from build123d import *

# Parameters (mm, degrees)
ESQUISSE1_W             = 7
ESQUISSE1_H             = 7
BOSS_EXTRU_1_DEPTH      = 8.4
CHANFREIN1_SIZE         = 2
CHANFREIN1_SIZE2        = 0.727940469
ESQUISSE2_R             = 1.25
ENL_V_MAT_EXTRU_1_DEPTH = 4


with BuildPart() as part:
    # Esquisse1 → Boss.-Extru.1 (new body)
    with BuildSketch(Plane(origin=(0, 0, 0), x_dir=(1, 0, 0), z_dir=(0, 1, 0))):
        with Locations((3.5, -3.5)):
            Rectangle(ESQUISSE1_W, ESQUISSE1_H)
    extrude(amount=BOSS_EXTRU_1_DEPTH)

    # Chanfrein1
    chanfrein1_edges = [part.edges().sort_by_distance(p)[0] for p in [
        (0, 8.4, 3.5),
    ]]
    chanfrein1_side = [part.faces().sort_by_distance(p)[0] for p in [
        (0, 4.2, 3.5),
    ]]
    chamfer(chanfrein1_edges, length=CHANFREIN1_SIZE, length2=CHANFREIN1_SIZE2, reference=chanfrein1_side[0])

    # Esquisse2 → Enlèv. mat.-Extru.1 (cut)
    with BuildSketch(Plane(origin=(0, 8.4, 0), x_dir=(1, 0, 0), z_dir=(0, 1, 0))):
        with Locations(Location((3.5, -1.7, 0), (0, 0, 270))):
            Circle(ESQUISSE2_R)
        with Locations(Location((3.5, -5.3, 0), (0, 0, 270))):
            Circle(ESQUISSE2_R)
    extrude(amount=-ENL_V_MAT_EXTRU_1_DEPTH, mode=Mode.SUBTRACT)


solid = part.part
Build history of the part. All positions in model axes, mm. A direction names the side the tool comes from. Coordinates: 2 decimals unless noted, no trailing zeros. Write each loop counter-clockwise with the first axis right and the second up, starting at its lowest first coordinate (ties: lowest second). Pieces come first, ordered by that corner, then holes.
(1) 3-axis set-ups, long thin cutter, end or side, ignore diameter. For faces 1 (the cylindrical face through (2.74, 6.43, 0.71)), 2 (the flat face through (3, 0, 3)): which of +Z, -Z, +X, -X, +Y, -Y reach the whole face in a straight line?
(2) Mould opens along X. For faces 3 (the flat face through (4, 4.4, 5)), 4 (the flat face through (7, 4, 4)), 5 (the flat face through (3.8, 8.4, 3.5)) say: pulls with the +X half, pulls with the -X half, needs draft (parallel to the pull), parting line crosses it, or undercut.
(3) Cut at D-D on z = 2.25. List the corners of the cut face in (x, y).
(4) Drill centre lines: line 1 (Z direction, x = 3, y = 7); line 2 (X direction, y = 5.75, z = 1.7); line 3 (Y direction, x = 2.75, z = 2.5). Where is each one in solid material? Low to high.
(5) Cut at A-A on y = 6. List the corners of the cut face in (x, z), and give its area (3 significant figures).
(6) Cut at B-B on z = 5.3. List the corners of the cut face in (x, y), and give its area (3 significant figures).
(7) Pin check, flat tip, straight feed: pin 1 Ø1.5 at (x, z) = (3.5, 5.3) entering from +Y. Stop position of the tip, or through.
(8) Cut at C-C on x = 3.5. List the corners of the cut face in (y, z), and give its area (3 significant figures).
Working result:
1. face 1: +Y
1. face 2: +Z, -Z, +X, -X, -Y
2. face 3: undercut
2. face 4: pulls with the +X half
2. face 5: needs draft
3. outline: (0, 0) - (7, 0) - (7, 8.4) - (4.62, 8.4) - (4.62, 4.4) - (2.38, 4.4) - (2.38, 8.4) - (0.73, 8.4) - (0, 6.4) - close
4. line 1: z = 0 to 0.55, 2.85 to 4.15, 6.45 to 7
4. line 2: x = 0 to 2.25, 4.75 to 7
4. line 3: y = 0 to 4.4
5. outline: (0, 0) - (7, 0) - (7, 7) - (0, 7) - close; hole circle Ø2.5 at (3.5, 1.7); hole circle Ø2.5 at (3.5, 5.3)
5. area: 39.2 mm2
6. outline: (0, 0) - (7, 0) - (7, 8.4) - (4.75, 8.4) - (4.75, 4.4) - (2.25, 4.4) - (2.25, 8.4) - (0.73, 8.4) - (0, 6.4) - close
6. area: 48.1 mm2
7. pin 1: stops at y = 4.4
8. outline: (0, 0) - (8.4, 0) - (8.4, 0.45) - (4.4, 0.45) - (4.4, 2.95) - (8.4, 2.95) - (8.4, 4.05) - (4.4, 4.05) - (4.4, 6.55) - (8.4, 6.55) - (8.4, 7) - (0, 7) - close
8. area: 38.8 mm2
